from build123d import *

# Parameters (mm, degrees)
SKETCH1_W           = 175
SKETCH1_H           = 63
BOSS_EXTRUDE1_DEPTH = 2.5
SKETCH2_R           = 1.75
CUT_EXTRUDE1_DEPTH  = 94.131627281
SKETCH3_R           = 7.5
CUT_EXTRUDE2_DEPTH  = 94.131627281
FILLET1_R           = 5
SKETCH4_R           = 1.75
CUT_EXTRUDE3_DEPTH  = 94.131627281


with BuildPart() as part:
    # Sketch1 → Boss-Extrude1 (new, symmetric)
    with BuildSketch(Plane(origin=(0, 0, 0), x_dir=(1, 0, 0), z_dir=(0, 1, 0))):
        Rectangle(SKETCH1_W, SKETCH1_H)
    extrude(amount=BOSS_EXTRUDE1_DEPTH, both=True)

    # Sketch2 → Cut-Extrude1 (cut, through all)
    with BuildSketch(Plane(origin=(0, 2.5, 0), x_dir=(1, 0, 0), z_dir=(0, 1, 0))):
        with Locations(Location((-82.5, 10, 0), (0, 0, 270))):
            Circle(SKETCH2_R)
        with Locations(Location((-62.5, 10, 0), (0, 0, 270))):
            Circle(SKETCH2_R)
        with Locations(Location((-54.5, 27, 0), (0, 0, 270))):
            Circle(SKETCH2_R)
        with Locations(Location((-35.37, 25.2, 0), (0, 0, 270))):
            Circle(SKETCH2_R)
        with Locations(Location((-29.24, 21.5, 0), (0, 0, 270))):
            Circle(SKETCH2_R)
        with Locations(Location((22.38, 25.2, 0), (0, 0, 270))):
            Circle(SKETCH2_R)
        with Locations(Location((16.26, 21.5, 0), (0, 0, 270))):
            Circle(SKETCH2_R)
        with Locations(Location((41.5, 27, 0), (0, 0, 270))):
            Circle(SKETCH2_R)
        with Locations(Location((41.5, -27, 0), (0, 0, 90))):
            Circle(SKETCH2_R)
        with Locations(Location((22.38, -25.2, 0), (0, 0, 90))):
            Circle(SKETCH2_R)
        with Locations(Location((16.26, -21.5, 0), (0, 0, 90))):
            Circle(SKETCH2_R)
        with Locations(Location((-29.24, -21.5, 0), (0, 0, 90))):
            Circle(SKETCH2_R)
        with Locations(Location((-35.37, -25.2, 0), (0, 0, 90))):
            Circle(SKETCH2_R)
        with Locations(Location((-62.5, -10, 0), (0, 0, 90))):
            Circle(SKETCH2_R)
        with Locations(Location((-54.5, -27, 0), (0, 0, 90))):
            Circle(SKETCH2_R)
        with Locations(Location((-82.5, -10, 0), (0, 0, 90))):
            Circle(SKETCH2_R)
    extrude(amount=-CUT_EXTRUDE1_DEPTH, mode=Mode.SUBTRACT)

    # Sketch3 → Cut-Extrude2 (cut, through all)
    with BuildSketch(Plane(origin=(0, 2.5, 0), x_dir=(1, 0, 0), z_dir=(0, 1, 0))):
        with BuildLine():
            ThreePointArc((-10.239221922, 19.791545875), (-9.505365031, 18.85426183), (-8.368903032, 18.5))
            Line((-8.368903032, 18.5), (8.368903032, 18.5))
            ThreePointArc((8.368903032, 18.5), (9.505365031, 18.85426183), (10.239221922, 19.791545875))
            Line((10.239221922, 19.791545875), (11.224070407, 22.391545875))
            ThreePointArc((11.224070407, 22.391545875), (10.999489687, 24.236461999), (9.353751517, 25.1))
            Line((9.353751517, 25.1), (-9.353751517, 25.1))
            ThreePointArc((-9.353751517, 25.1), (-10.999489687, 24.236461999), (-11.224070407, 22.391545875))
            Line((-11.224070407, 22.391545875), (-10.239221922, 19.791545875))
        make_face()
        with BuildLine():
            Line((45.85, -8.489291496), (45.85, 8.489291496))
            ThreePointArc((45.85, 8.489291496), (45.066439614, 9.465587503), (43.943692213, 8.911909758))
            Line((43.943692213, 8.911909758), (40.182140708, 0.845236523))
            ThreePointArc((40.182140708, 0.845236523), (39.994756282, 0), (40.182140708, -0.845236523))
            Line((40.182140708, -0.845236523), (43.943692213, -8.911909758))
            ThreePointArc((43.943692213, -8.911909758), (45.066439614, -9.465587503), (45.85, -8.489291496))
        make_face()
        with BuildLine():
            Line((-9.353751517, -25.1), (9.353751517, -25.1))
            ThreePointArc((9.353751517, -25.1), (10.999489687, -24.236461999), (11.224070407, -22.391545875))
            Line((11.224070407, -22.391545875), (10.239221922, -19.791545875))
            ThreePointArc((10.239221922, -19.791545875), (9.505365031, -18.85426183), (8.368903032, -18.5))
            Line((8.368903032, -18.5), (-8.368903032, -18.5))
            ThreePointArc((-8.368903032, -18.5), (-9.505365031, -18.85426183), (-10.239221922, -19.791545875))
            Line((-10.239221922, -19.791545875), (-11.224070407, -22.391545875))
            ThreePointArc((-11.224070407, -22.391545875), (-10.999489687, -24.236461999), (-9.353751517, -25.1))
        make_face()
        with BuildLine():
            Line((57.5, -15.4), (57.5, 15.4))
            ThreePointArc((57.5, 15.4), (55.9, 17), (54.3, 15.4))
            Line((54.3, 15.4), (54.3, -15.4))
            ThreePointArc((54.3, -15.4), (55.9, -17), (57.5, -15.4))
        make_face()
        with Locations(Location((0, 0, 0), (0, 0, 270))):
            Circle(SKETCH3_R)
    extrude(amount=-CUT_EXTRUDE2_DEPTH, mode=Mode.SUBTRACT)

    # Fillet1
    fillet1_edges = [part.edges().sort_by_distance(p)[0] for p in [
        (87.5, 0, 31.5),
        (-87.5, 0, 31.5),
        (-87.5, 0, -31.5),
        (87.5, 0, -31.5),
    ]]
    fillet(fillet1_edges, radius=FILLET1_R)

    # Sketch4 → Cut-Extrude3 (cut, through all)
    with BuildSketch(Plane(origin=(0, 2.5, 0), x_dir=(1, 0, 0), z_dir=(0, 1, 0))):
        with Locations(Location((72.5, 25, 0), (0, 0, 270))):
            Circle(SKETCH4_R)
        with Locations(Location((72.5, -25, 0), (0, 0, 270))):
            Circle(SKETCH4_R)
    extrude(amount=-CUT_EXTRUDE3_DEPTH, mode=Mode.SUBTRACT)


solid = part.part
Could you check a few things on this model? Use its own coordinates, in mm. A direction names the side the tool comes from. Coordinates: 2 decimals unless noted, no trailing zeros. Loops run counter-clockwise (first coordinate to the right, second up) from the corner with the lowest first, then second, coordinate; pieces in that order, holes last.
1. For faces 5 (the face through (-1, 0, 31.5)), 6 (the face through (0, 0, 18.5)), which set-ups out of +Z, -Z, +X, -X, +Y, -Y let a thin tool reach every point of the face, with its end or its side?
2. We'd pull the mould along Z, two halves only. Please class faces 1 (the face through (-86.07, 0.04, 30)), 2 (the face through (-1, -2.5, -14)), 3 (the face through (42.09, 0.04, -4.94)), 4 (the face through (86, -0.04, -30.07)): released by +Z, released by -Z, zero draft, split by the parting line, or undercut.
3. For P1, Ø3, axis at x = -54.5, z = -27, coming from the +Y side, with a flat end and sliding along its axis, tell me the tip position at first contact or that it passes through.
4. Imagine slicing it at B-B (z = 3). Please give me the cut outline in (x, y).
5. Imagine slicing it at D-D (y = 1.4). Give the number of separate pieces and of enclosed holes in the cut face, and give its area (3 significant figures).
6. Imagine slicing it at A-A (x = -4.5). Please give me the cut outline in (y, z).
7. I need wall thicknesses on L1, parallel to X at y = -0.4, z = 25.2; L2, parallel to X at y = 0.9, z = 27; L3, parallel to X at y = 0, z = 10. Which ranges of each line are inside material? Lowest first, please.
8. Imagine slicing it at C-C (x = -29.24). Please give me the cut outline in (y, z), and give its area (3 significant figures).
Computed values:
1. face 5: +Z, +X, -X, +Y, -Y
1. face 6: +Y, -Y
2. face 1: released by +Z
2. face 2: zero draft
2. face 3: undercut
2. face 4: released by -Z
3. P1: passes through
4. outline: (-87.5, -2.5) - (-6.87, -2.5) - (-6.87, 2.5) - (-87.5, 2.5) - close; (6.87, -2.5) - (41.19, -2.5) - (41.19, 2.5) - (6.87, 2.5) - close; (45.85, -2.5) - (54.3, -2.5) - (54.3, 2.5) - (45.85, 2.5) - close; (57.5, -2.5) - (87.5, -2.5) - (87.5, 2.5) - (57.5, 2.5) - close
5. separate pieces: 1
5. enclosed holes: 23
5. area: 10,200 mm2
6. outline: (-2.5, -31.5) - (2.5, -31.5) - (2.5, -25.1) - (-2.5, -25.1) - close; (-2.5, -18.5) - (2.5, -18.5) - (2.5, -6) - (-2.5, -6) - close; (-2.5, 6) - (2.5, 6) - (2.5, 18.5) - (-2.5, 18.5) - close; (-2.5, 25.1) - (2.5, 25.1) - (2.5, 31.5) - (-2.5, 31.5) - close
7. L1: x = -87.5 to -37.12, -33.62 to 20.63, 24.13 to 70.76, 74.24 to 87.5
7. L2: x = -87.47 to -56.25, -52.75 to 39.75, 43.25 to 87.47
7. L3: x = -87.5 to -84.25, -80.75 to -64.25, -60.75 to 54.3, 57.5 to 87.5
8. outline: (-2.5, -31.5) - (2.5, -31.5) - (2.5, -23.25) - (-2.5, -23.25) - close; (-2.5, -19.75) - (2.5, -19.75) - (2.5, 19.75) - (-2.5, 19.75) - close; (-2.5, 23.25) - (2.5, 23.25) - (2.5, 31.5) - (-2.5, 31.5) - close
8. area: 280 mm2
